For this review, use the dimensioned drawing (mm, ordinates from the lowest corner) and the shaded views. Coordinates: 2 decimals unless noted, no trailing zeros. Order: outer loops, then holes, each group sorted by start corner. A loop starts at its lowest first (then second) coordinate and runs counter-clockwise, first axis right, second up. Notation, with made-up numbers: M 17.5,64 L 34.5,64 A9 ccw 34.5,78 Z; hole C -5,37 d1. An arc over 180 degrees is marked long. Answer as CSV lines item,"result". Start each with the question number.
Q1. Consider section D-D on y = 4.5. Write out the cut boundary in (x, z) (1 decimal).
Q2. Wall thickness on L1, parallel to Y at x = 1.6, z = 13.25 (1 decimal); L2, parallel to Y at x = 0.5, z = 12.75 (1 decimal); L3, parallel to Z at x = 0.75, y = 23: over which ranges is each line inside the solid? List them lowest first. Write a range as [from, to].
Q3. Consider section C-C on x = 1.7. State how many separate pieces and enclosed holes the cut face has, and give its area (3 significant figures).
Q4. Consider section A-A on z = 11. Write out the cut boundary in (x, y).
Q5. For P1, Ø2.5, axis at y = 12.65, z = 20.59, coming from the +X side; P2, Ø1.5, axis at y = 11.5, z = 20.5, coming from the -X side, all flat-tipped, find the tip position at first contact; note any pin that passes through.
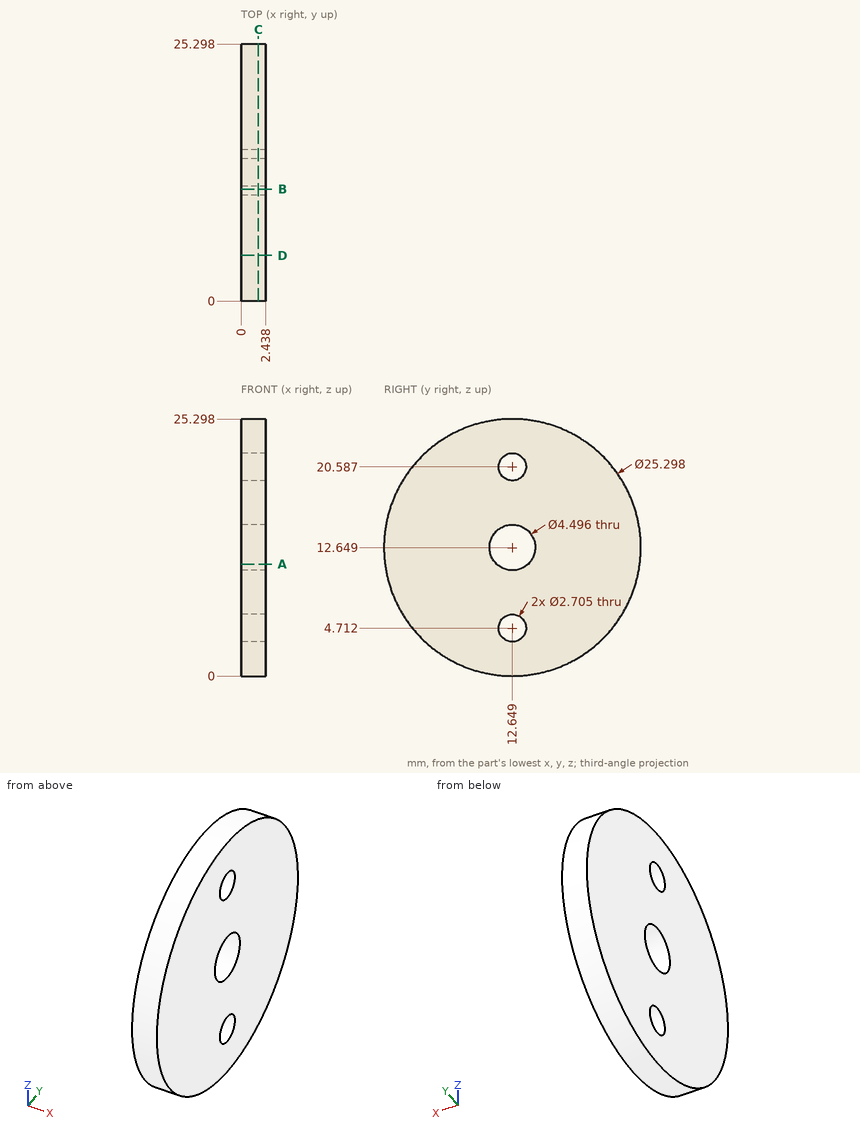
Evaluation:
1,outline,"M 0,3 L 2.4,3 L 2.4,22.3 L 0,22.3 Z"
2,L1,"y = [0, 10.5], [14.8, 25.3]"
2,L2,"y = [0, 10.4], [14.9, 25.3]"
2,L3,"z = [5.38, 19.92]"
3,separate pieces,"1"
3,enclosed holes,"3"
3,area,"475 mm²"
4,outline,"M 0,0.11 L 2.44,0.11 L 2.44,11.12 L 0,11.12 Z; M 0,14.18 L 2.44,14.18 L 2.44,25.19 L 0,25.19 Z"
5,P1,"passes through"
5,P2,"stops at x = 0"
